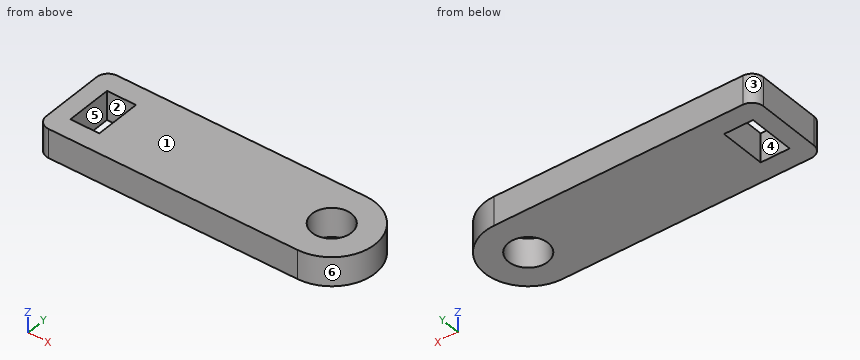
Autodesk Inventor part; units mm, degrees
ref_plane "YZ Plane" through (0, 0, 0) normal (1, 0, 0) x (0, 1, 0)
ref_plane "XZ Plane" through (0, 0, 0) normal (0, 1, 0) x (-1, 0, 0)
ref_plane "XY Plane" through (0, 0, 0) normal (0, 0, 1) x (1, 0, 0)
sketch "Skizze1" plane through (0, 0, 0) normal (0, 0, 1) x (1, 0, 0)
  line L0 (0, -24.15) -> (0, 24.15)
  line L1 (-77.25, 0) -> (33, 0)
  circle A0 centre (-15.5, 15.5) radius 1.75
  circle A1 centre (15.5, 15.5) radius 1.75
  circle A2 centre (-15.5, -15.5) radius 1.75
  circle A3 centre (15.5, -15.5) radius 1.75
  circle A4 centre (-16.5, 0) radius 11
  circle A5 centre (0, 0) radius 5.5
  circle A6 centre (-16.5, 0) radius 3.4
  arc A7 (-16.5, -7.5) -> (-16.5, 7.5) centre (-16.5, 0) ccw
  line L2 (-16.5, 7.5) -> (-36.5, 7.5)
  line L3 (-36.5, 7.5) -> (-61.5, 7.5)
  line L4 (-61.5, 7.5) -> (-61.5, -7.5)
  line L5 (-61.5, -7.5) -> (-16.5, -7.5)
  dimension "d0" = 3.5
  dimension "d1" = 15.5
  dimension "d2" = 15.5
  dimension "d3" = 22
  dimension "d4" = 16.5
  dimension "d5" = 11
  dimension "d6" = 6.8
  dimension "d7" = 15
  dimension "d10" = 15
  dimension "d11" = 45
extrude "Extrusion1" add sketch "Skizze1" along normal blind 5 contours A7 L5 A4 L1 A6 | L1 A6 A4 L2 A7 | A4 L1 L4 L3 L2 | L5 L4 L1 A4
sketch "Skizze3" plane through (0, 0, 0) normal (0, 0, -1) x (-1, 0, 0)
  circle A0 centre (16.5, 0) radius 3.4
  arc A1 (16.5, 7.5) -> (16.5, -7.5) centre (16.5, 0) ccw
  line L0 (16.5, -7.5) -> (61.5, -7.5)
  line L1 (61.5, -7.5) -> (61.5, 7.5)
  line L2 (61.5, 7.5) -> (16.5, 7.5)
  line L3 (58.5, -4) -> (53.5, -4)
  line L4 (53.5, -4) -> (53.5, 4)
  line L5 (53.5, 4) -> (58.5, 4)
  line L6 (58.5, 4) -> (58.5, -4)
  line L7 (73.8, 0) -> (-12.3, 0)
  point P0 (0, 0)
  dimension "d17" = 5
  dimension "d18" = 8
  dimension "d19" = 3
extrude "Extrusion3" cut sketch "Skizze3" against normal blind 5 contours L7 L6 L3 L4 | L4 L5 L6 L7
fillet "Rundung1" radius 2 2 edges at (-61.5, 7.5, 2.5) (-61.5, -7.5, 2.5)
properties part number "Kugellager-Schieber-Seite_M8Gewinde" material "ABS-Kunststoff"
Geometry: final body of the model. Coordinates: model frame, mm. Face numbers are marked on the shaded views. A direction names the side the tool comes from. Give positions to 0.01 mm unless a question says otherwise; leave off trailing zeros. Order: outer loops, then holes, each group sorted by start corner. A loop starts at its lowest first (then second) coordinate and runs counter-clockwise, first axis right, second up. Notation, with made-up numbers: (10.5, 53.5) -> (21.5, 53.5) arc R25 cw to (21.5, 84.5) -> close; hole circle Ø4 at (13.5, -31). An arc over 180 degrees is marked (long way). Write each question's results on one line, items separated by ' | '. Start each with the question number.
1) Draft query along X for the marked faces 1, 2, 3 and 4. Return one class per face: pulls with the +X half, pulls with the -X half, needs draft (parallel to the pull), parting line crosses it, or undercut.
2) Section A-A (y = 0). Return loops of the section in (x, z).
3) Set-up query: the marked faces 5 and 6. Return all of +Z, -Z, +X, -X, +Y, -Y with unobstructed straight access to the full face (end or side cutting, diameter ignored); none if empty.
4) Section B-B (x = -57). Return loops of the section in (y, z).
5) Line query: line 1 (X direction, y = 0, z = 1.1); line 2 (Y direction, x = -16.5, z = 2.3); line 3 (Y direction, x = -57, z = 2.7). Output: solid intervals per line, ascending. Write a range as from..to.
6) Section D-D (y = -6.25). Return loops of the section in (x, z).
7) Section C-C (z = 4.2). Return loops of the section in (x, y).
Calculated:
1) face 1: needs draft | face 2: undercut | face 3: pulls with the -X half | face 4: undercut
2) outline: (-61.5, 0) -> (-58.5, 0) -> (-58.5, 5) -> (-61.5, 5) -> close; (-53.5, 0) -> (-19.9, 0) -> (-19.9, 5) -> (-53.5, 5) -> close; (-13.1, 0) -> (-9, 0) -> (-9, 5) -> (-13.1, 5) -> close
3) face 5: +Z, -Z | face 6: +Z, -Z, +X
4) outline: (-7.5, 0) -> (-4, 0) -> (-4, 5) -> (-7.5, 5) -> close; (4, 0) -> (7.5, 0) -> (7.5, 5) -> (4, 5) -> close
5) line 1: -61.5..-58.5, -53.5..-19.9, -13.1..-9 | line 2: -7.5..-3.4, 3.4..7.5 | line 3: -7.5..-4, 4..7.5
6) outline: (-61.35, 0) -> (-12.35, 0) -> (-12.35, 5) -> (-61.35, 5) -> close
7) outline: (-61.5, -5.5) arc R2 ccw to (-59.5, -7.5) -> (-16.5, -7.5) arc R7.5 ccw to (-16.5, 7.5) -> (-59.5, 7.5) arc R2 ccw to (-61.5, 5.5) -> close; hole (-58.5, -4) -> (-53.5, -4) -> (-53.5, 4) -> (-58.5, 4) -> close; hole circle Ø6.8 at (-16.5, 0)
